from build123d import *

# Parameters (mm, degrees)
F0_R     = 12.7
F1_DEPTH = 76.2


with BuildPart() as f1:
    # F0 (on Top) → F1 (new body)
    with BuildSketch(Plane.XY):
        with BuildLine():
            ThreePointArc((17.607051, -7.272844), (18.685781, -3.707302), (19.05, 0))
            ThreePointArc((19.05, 0), (18.685781, 3.707302), (17.607051, 7.272844))
            ThreePointArc((17.607051, 7.272844), (10.177085, 11.202116), (5.555008, 18.222085))
            ThreePointArc((5.555008, 18.222085), (0, 19.05), (-5.555008, 18.222085))
            ThreePointArc((-5.555008, 18.222085), (-10.177085, 11.202116), (-17.607051, 7.272844))
            ThreePointArc((-17.607051, 7.272844), (-19.05, 0), (-17.607051, -7.272844))
            ThreePointArc((-17.607051, -7.272844), (-10.177085, -11.202116), (-5.555008, -18.222085))
            ThreePointArc((-5.555008, -18.222085), (0, -19.05), (5.555008, -18.222085))
            ThreePointArc((5.555008, -18.222085), (10.177085, -11.202116), (17.607051, -7.272844))
        make_face()
        Circle(F0_R, mode=Mode.SUBTRACT)
    extrude(amount=F1_DEPTH)


solid = f1.part
Work out the finished part from the listing and answer in its coordinate system (mm). Coordinates: 2 decimals unless noted, no trailing zeros. Order: outer loops, then holes, each group sorted by start corner. A loop starts at its lowest first (then second) coordinate and runs counter-clockwise, first axis right, second up. Notation, with made-up numbers: (-26.75, 19) - (-21.75, 19) arc R19 ccw to (-21.75, 24) - close; hole circle Ø3 at (-3, 34.25). An arc over 180 degrees is marked (long way). Put each result on its own line as item: value. Start each with the question number.
1) Flat-ended cylindrical pins translate along their axes: pin 1 (10 mm diameter, centred on x = 4, y = 7.5, fed in from -Z); pin 2 (1 mm diameter, centred on x = -6.5, z = 51.5, fed in from -Y); pin 3 (4 mm diameter, centred on y = 6.5, z = 35, fed in from +X); pin 4 (5 mm diameter, centred on x = -13, z = 60.5, fed in from +Y). Find the tip coordinate at first contact, or state that the pin passes through.
2) Find section C-C (z = 59.5). Give the vertices of the cut face in (x, y) (3 decimals), plus the area to 3 significant figures.
3) Find the intervals of material crossed by line 1 (X direction, y = -4.5, z = 35.5); line 2 (X direction, y = 11.5, z = 25.5); line 3 (Y direction, x = -8.5, z = 67.5), in increasing order. Write a range as from..to.
4) Find section A-A (x = 0). Give the vertices of the cut face in (y, z).
5) For a pull along Y with two mould halves and no side action, classify faces 1 (the flat face through (-9, -10, 0)), 2 (the cylindrical face through (-2.75, -12.4, 37.57)), 3 (the cylindrical face through (-10.27, -11.12, 37.57)) as released by +Y, released by -Y, zero draft, split by the parting line, or undercut.
6) Find section B-B (y = -5.5). Give the vertices of the cut face in (x, z).
Results list:
1. pin 1: stops at z = 0
1. pin 2: stops at y = -17.07
1. pin 3: stops at x = 18.51
1. pin 4: stops at y = 10.92
2. outline: (-17.607, -7.273) arc R16.918 cw to (-5.555, -18.222) arc R19.05 ccw to (5.555, -18.222) arc R16.918 cw to (17.607, -7.273) arc R19.05 ccw to (17.607, 7.273) arc R16.918 cw to (5.555, 18.222) arc R19.05 ccw to (-5.555, 18.222) arc R16.918 cw to (-17.607, 7.273) arc R19.05 ccw to start; hole circle Ø25.4 at (0, 0)
2. area: 461 mm^2
3. line 1: x = -18.51..-11.88, 11.88..18.51
3. line 2: x = -9.86..-5.39, 5.39..9.86
3. line 3: y = -12.96..-9.44, 9.44..12.96
4. outline: (-19.05, 0) - (-12.7, 0) - (-12.7, 76.2) - (-19.05, 76.2) - close; (12.7, 0) - (19.05, 0) - (19.05, 76.2) - (12.7, 76.2) - close
5. face 1: zero draft
5. face 2: undercut
5. face 3: released by -Y
6. outline: (-18.24, 0) - (-11.45, 0) - (-11.45, 76.2) - (-18.24, 76.2) - close; (11.45, 0) - (18.24, 0) - (18.24, 76.2) - (11.45, 76.2) - close
